The drawing under review shows one solid part. Ordinate dimensions are in mm from its lowest x, y, z. A direction names the side the tool comes from. Coordinates: 2 decimals unless noted, no trailing zeros. Loops run counter-clockwise (first coordinate to the right, second up) from the corner with the lowest first, then second, coordinate; pieces in that order, holes last. Notation, with made-up numbers: (54, -22) - (91, -22) arc R19 ccw to (91, -11) - close; hole circle Ø10 at (17, -6). An arc over 180 degrees is marked (long way). Use one line per item in the form item = value. Start each with the question number.
1. For pin 1 Ø5 at (y, z) = (36.5, 39) entering from +X; pin 2 Ø5 at (y, z) = (38, 24.5) entering from -X, all flat-tipped, find the tip position at first contact; note any pin that passes through.
2. Add section A-A on y = 14.5. Give the boundary of the cut face in (x, z), and give its area (3 significant figures).
3. Add section B-B on z = 118. Give the boundary of the cut face in (x, y), and give its area (3 significant figures).
4. To check wall thickness, follow probe 1 along Y at (x, z) = (61.5, 22); probe 2 along X at (y, z) = (12.5, 79.5). State the ranges of each line that lie inside material, in increasing order.
5. Machinability: for the marked faces 1, 2 and 3, which of the approach directions +Z, -Z, +X, -X, +Y, -Y give a long, thin tool a straight path to every point of the face, cutting with its end or side? Answer none if there is none.
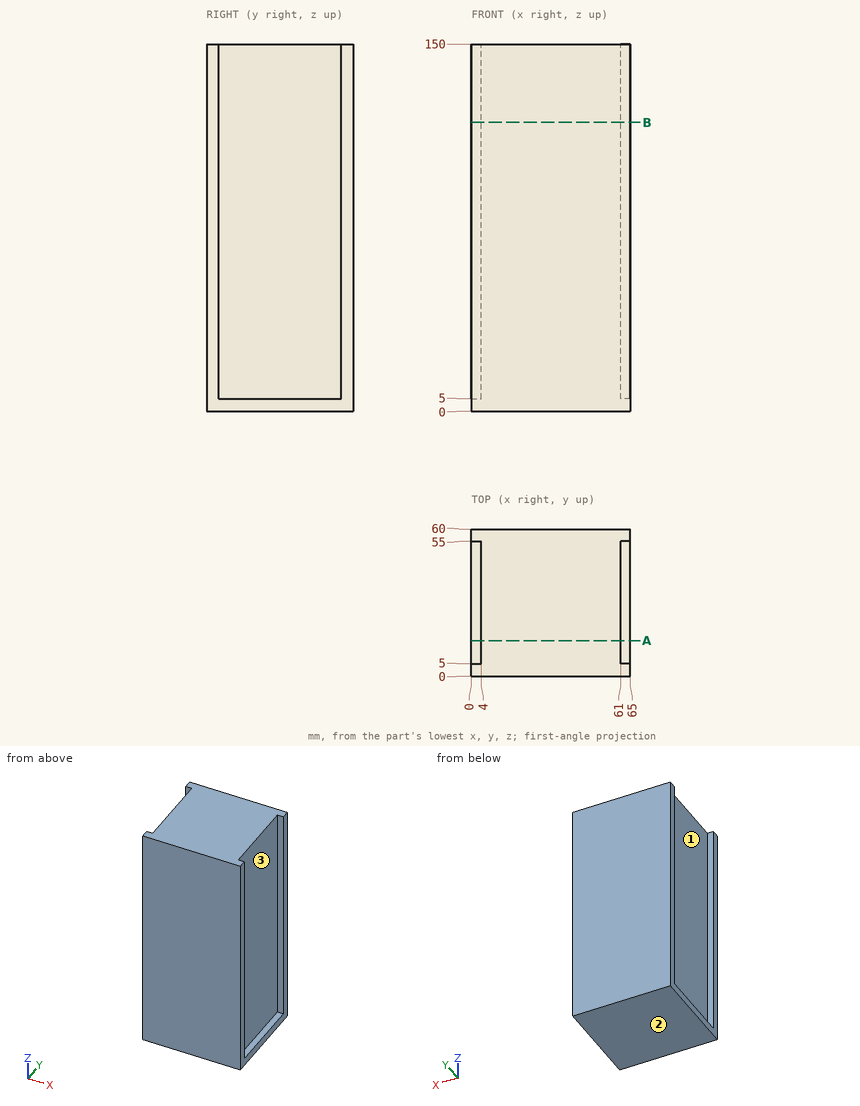
Conclusion:
q1.pin_1 = 61
q1.pin_2 = 4
q2.outline = (0, 0) - (65, 0) - (65, 5) - (61, 5) - (61, 150) - (4, 150) - (4, 5) - (0, 5) - close
q2.area = 8,590 mm^2
q3.outline = (0, 0) - (65, 0) - (65, 5) - (61, 5) - (61, 55) - (65, 55) - (65, 60) - (0, 60) - (0, 55) - (4, 55) - (4, 5) - (0, 5) - close
q3.area = 3,500 mm^2
q4.probe_1 = 0 to 5, 55 to 60
q4.probe_2 = 4 to 61
q5.face_1 = +Z, -X
q5.face_2 = -Z, +X, -X, +Y, -Y
q5.face_3 = +Z, +X
